Verification items for the finished model (mm, model axes). Round coordinates to 2 decimals unless told otherwise and drop trailing zeros. Write each loop counter-clockwise with the first axis right and the second up, starting at its lowest first coordinate (ties: lowest second). Pieces come first, ordered by that corner, then holes. Notation, with made-up numbers: (-25.75, 63) -> (-11.75, 63) arc R13 ccw to (-11.75, 68) -> close; hole circle Ø4 at (67, 62.25). An arc over 180 degrees is marked (long way). Answer as a JSON object with one key per item and string values. Group by question number.
(1) Sectioned sample at A-A on z = 0.5. Record the cut outline in (x, y), and give its area (3 significant figures).
(2) Sectioned sample at D-D on y = 510. Record the cut outline in (x, z).
(3) Scan lines: L1, parallel to Y at x = 30, z = 1.1; L2, parallel to X at y = 369.15, z = 1.2; L3, parallel to Z at x = 23.5, y = 427. Record each from-to range of solid material in increasing order. Write a range as from..to.
(4) Sectioned sample at C-C on y = 470. Record the cut outline in (x, z).
(5) Gauge pin test, flat ends, axial feed: pin 1 Ø3.5 at (x, y) = (37.5, 537) entering from +Z; pin 2 Ø2 at (x, y) = (98.04, 523.1) entering from +Z. Record the tip position at first contact, or that the pin passes through.
```python
from build123d import *

# Parameters (mm, degrees)
EXTRUDE1_DEPTH     = 1.5875
EXTRUDE3_DEPTH     = 2.5875
SKETCH3_R          = 1.7272
EXTRUDE2_DEPTH     = 2.5875
CUT_EXTRUDE1_DEPTH = 0.005


with BuildPart() as part:
    # Sketch1 → Extrude1 (new body)
    with BuildSketch(Plane(origin=(0, 0, 0), x_dir=(-1, 0, 0), z_dir=(0, 0, -1))):
        Polygon((-139.214433641, 524.126541463), (-52.060002376, 196), (52.060002376, 196), (139.214433641, 524.126541463), (0, 542.3), align=None)
    extrude(amount=-EXTRUDE1_DEPTH)

    # Sketch5 → Extrude3 (cut, through all)
    with BuildSketch(Plane.XY.offset(1.5875)):
        Polygon((-138.475953663, 521.346248167), (-111.862580021, 527.697132275), (-139.214433641, 524.126541463), align=None)
        Polygon((139.214433641, 524.126541463), (138.475953663, 521.346248167), (111.862580021, 527.697132275), align=None)
    extrude(amount=-EXTRUDE3_DEPTH, mode=Mode.SUBTRACT)

    # Sketch3 → Extrude2 (cut, through all)
    with BuildSketch(Plane.XY.offset(1.5875)):
        with Locations((-98.040924265, 523.097573518)):
            Circle(SKETCH3_R)
        with Locations((-30, 202.35)):
            Circle(SKETCH3_R)
        with Locations(Location((30, 202.35, 0), (0, 0, 180))):  # turned: the seam where the file's is
            Circle(SKETCH3_R)
        with Locations(Location((98.040924265, 523.097573518, 0), (0, 0, 180))):  # turned: the seam where the file's is
            Circle(SKETCH3_R)
        with Locations((0, 369.15)):
            Circle(SKETCH3_R)
    extrude(amount=-EXTRUDE2_DEPTH, mode=Mode.SUBTRACT)

    # Sketch4 → Cut-Extrude1 (cut)
    with BuildSketch(Plane.XY.offset(1.5875)):
        with BuildLine():
            Line((110.847856253, 417.329597278), (107.587625187, 405.055197358))
            ThreePointArc((107.587625187, 405.055197358), (0, 419.1), (-107.587625187, 405.055197358))
            Line((-107.587625187, 405.055197358), (-110.847856253, 417.329597278))
            ThreePointArc((-110.847856253, 417.329597278), (0, 431.8), (110.847856253, 417.329597278))
        make_face()
        Polygon((-93.921186267, 530.039254187), (-93.5283394, 527.627083961), (-78.723393901, 530.038222445), (-79.039941137, 531.981895365), align=None)
        Polygon((27.790346618, 538.672167032), (27.559054717, 535.14333454), (42.526938566, 534.162287602), (42.695003931, 536.726469559), align=None)
        Polygon((-131.361910987, 525.151632692), (-130.105913895, 519.817603751), (-115.505225018, 523.255609615), (-116.411244397, 527.10333635), align=None)
    extrude(amount=-CUT_EXTRUDE1_DEPTH, mode=Mode.SUBTRACT)


solid = part.part
```
Computed values:
{
 "1": {"outline": "(-138.48, 521.35) -> (-52.06, 196) -> (52.06, 196) -> (138.48, 521.35) -> (111.86, 527.7) -> (0, 542.3) -> (-111.86, 527.7) -> close; hole circle Ø3.45 at (-98.04, 523.1); hole circle Ø3.45 at (-30, 202.35); hole circle Ø3.45 at (0, 369.15); hole circle Ø3.45 at (30, 202.35); hole circle Ø3.45 at (98.04, 523.1)", "area": "65,200 mm2"},
 "2": {"outline": "(-135.46, 0) -> (135.46, 0) -> (135.46, 1.59) -> (-135.46, 1.59) -> close"},
 "3": {"L1": "196..200.62, 204.08..538.38", "L2": "-98.05..-1.73, 1.73..98.05", "L3": "0..1.58"},
 "4": {"outline": "(-124.84, 0) -> (124.84, 0) -> (124.84, 1.59) -> (-124.84, 1.59) -> close"},
 "5": {"pin 1": "z = 1.58", "pin 2": "through"}
}
